Part print with two shaded views. Sizes in mm from the minimum x, y, z corner. Give positions to 0.01 mm unless a question says otherwise; leave off trailing zeros. Write each loop counter-clockwise with the first axis right and the second up, starting at its lowest first coordinate (ties: lowest second). Pieces come first, ordered by that corner, then holes. Notation, with made-up numbers: (16.5, 4.5) -> (45.5, 4.5) arc R23 cw to (45.5, 29.5) -> close; hole circle Ø6 at (57.25, 30). An arc over 180 degrees is marked (long way). Answer as a JSON object with one key per item and string values.
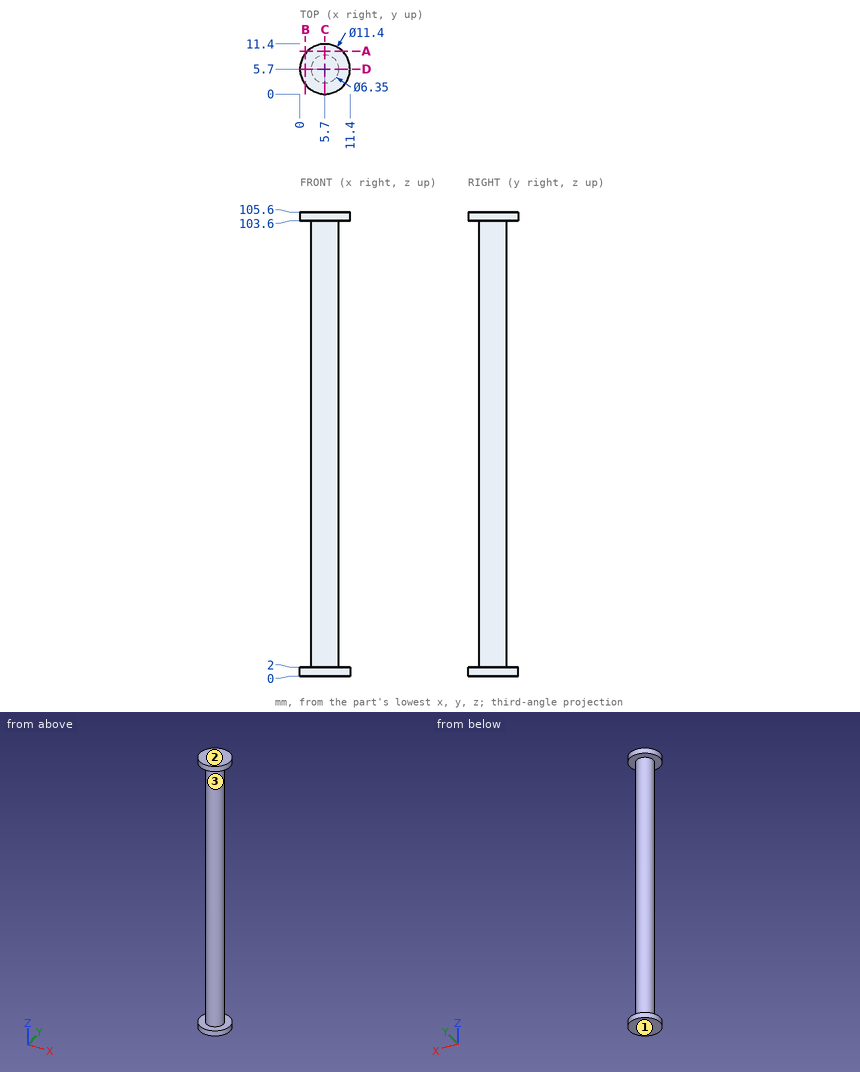
1) Slice it at C-C (x = 5.7). List the corners of the cut face in (y, z) (3 decimals).
Model answer:
{"outline": "(0, 0) -> (11.4, 0) -> (11.4, 2) -> (8.875, 2) -> (8.875, 103.6) -> (11.4, 103.6) -> (11.4, 105.6) -> (0, 105.6) -> (0, 103.6) -> (2.525, 103.6) -> (2.525, 2) -> (0, 2) -> close"}
2) Mould opens along Z. For the marked faces 1, 2 and 3 say: released by +Z, released by -Z, zero draft, split by the parting line, or undercut.
Model answer:
{"face 1": "released by -Z", "face 2": "released by +Z", "face 3": "undercut"}
3) Wall check: probe 1 along Z at (x, y) = (9.5, 2); probe 2 along Y at (x, z) = (5.75, 92.5); probe 3 along X at (y, z) = (5, 80). Give the ranges that are in metal, low to high.
Model answer:
{"probe 1": "z = 0 to 2, 103.6 to 105.6", "probe 2": "y = 2.53 to 8.87", "probe 3": "x = 2.6 to 8.8"}
4) Pin check, flat tips, straight feed: pin 1 (6 mm diameter, centred on x = 10, z = 41.5, fed in from -Y); pin 2 (1.5 mm diameter, centred on y = 6.5, z = 62.5, fed in from +X); pin 3 (1.5 mm diameter, centred on y = 8.5, z = 51.5, fed in from -X). Stop position of each tip, or through.
Model answer:
{"pin 1": "stops at y = 2.8", "pin 2": "stops at x = 8.87", "pin 3": "stops at x = 3.28"}
5) Slice it at A-A (y = 9.75). List the corners of the cut face in (x, z).
Model answer:
{"outline": "(1.69, 0) -> (9.71, 0) -> (9.71, 2) -> (1.69, 2) -> close; (1.69, 103.6) -> (9.71, 103.6) -> (9.71, 105.6) -> (1.69, 105.6) -> close"}
6) Slice it at B-B (x = 1.25). List the corners of the cut face in (y, z), then the cut area to 3 significant figures.
Model answer:
{"outline": "(2.14, 0) -> (9.26, 0) -> (9.26, 2) -> (2.14, 2) -> close; (2.14, 103.6) -> (9.26, 103.6) -> (9.26, 105.6) -> (2.14, 105.6) -> close", "area": "28.5 mm2"}
